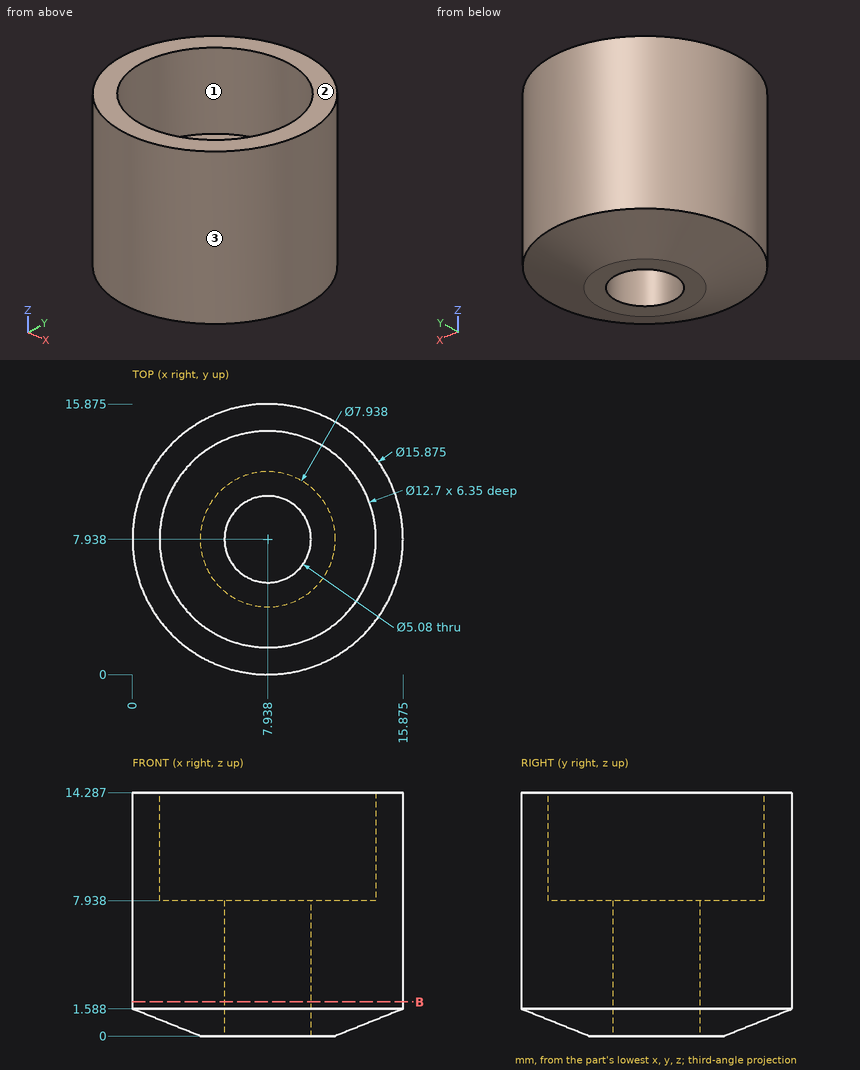
For this review, use the dimensioned drawing (mm, ordinates from the lowest corner) and the shaded views. Give positions to 0.01 mm unless a question says otherwise; leave off trailing zeros. Write each loop counter-clockwise with the first axis right and the second up, starting at its lowest first coordinate (ties: lowest second). Pieces come first, ordered by that corner, then holes. Notation, with made-up numbers: M 11,-32 L 38,-32 A5 cw 38,-23 Z; hole C 17.25,-1.5 d4. An arc over 180 degrees is marked long. Answer as a JSON object with one key per item and string values. Group by question number.
1) For line 1 along Y through (x, z) = (11.5, 8) (1 decimal); line 2 along X through (y, z) = (11, 12.75) (1 decimal); line 3 along Y through (x, z) = (9.25, 1.75) (1 decimal), list the stretches that pass through material, from the lowest coordinate up.
2) We need section B-B (z = 2). Give the boundary of the cut face in (x, y) (1 decimal).
3) Clearance check with flat-ended pins moving along their axes: pin 1 Ø1 at (y, z) = (13, 3) entering from +X; pin 2 Ø1 at (x, y) = (2.5, 3) entering from -Z; pin 3 Ø2 at (x, z) = (1.5, 3) entering from +Y; pin 4 Ø5 at (x, y) = (11.5, 5) entering from -Z. State where each tip first meets the part, or that it passes through.
4) Mouldability with a two-part tool opening along X and no side actions: class the marked faces 1, 2 and 3 as released by +X, released by -X, zero draft, split by the parting line, or undercut.
Answer key:
{
 "1": {"line 1": "y = 0.8 to 2.7, 13.2 to 15", "line 2": "x = 0.6 to 2.4, 13.5 to 15.3", "line 3": "y = 0.1 to 5.8, 10.1 to 15.8"},
 "2": {"outline": "C 7.9,7.9 d15.9; hole C 7.9,7.9 d5.1"},
 "3": {"pin 1": "stops at x = 14.43", "pin 2": "stops at z = 1.15", "pin 3": "stops at y = 13.72", "pin 4": "stops at z = 0"},
 "4": {"face 1": "undercut", "face 2": "zero draft", "face 3": "split by the parting line"}
}
